Geometry check sheet. Reference: the model listing, model coordinates, mm. Give positions to 0.01 mm unless a question says otherwise; leave off trailing zeros. Loops run counter-clockwise (first coordinate to the right, second up) from the corner with the lowest first, then second, coordinate; pieces in that order, holes last. Notation, with made-up numbers: (66.25, -1) - (94.25, -1) arc R27 ccw to (94.25, 15) - close; hole circle Ø2 at (59.5, 35.5). An arc over 180 degrees is marked (long way). Use a Markdown table: item, result. Add a question column.
1. Depth check by flat-ended pin: P1, Ø1.6, axis at y = 0, z = -1.5, coming from the -X side; P2, Ø0.7, axis at x = -155.5, y = -0.5, coming from the +Z side; P3, Ø1.6, axis at y = 0.5, z = 98, coming from the +X side. Enter the tip coordinate at first touch or a pass-through.
2. Cross-section at B-B on z = 135.5. Enter the section's corners in (x, y).
3. Cross-section at C-C on x = -15. Enter the section's corners in (y, z), and give its area (3 significant figures).
4. Material ranges on L1, parallel to X at y = 0.45, z = 144; L2, parallel to Z at x = -132, y = -0.95; L3, parallel to X at y = 1.35, z = 53, recorded low to high.
5. Cross-section at A-A on y = -0.8. Enter the section's corners in (x, z) (3 decimals).
from build123d import *

# Parameters (mm, degrees)
SKETCH1_W           = 314.32961264
SKETCH1_H           = 3.175
BOSS_EXTRUDE1_DEPTH = 200.60000012
CUT_EXTRUDE2_START  = -3.175
SKETCH5_W           = 2.286
SKETCH5_H           = 86.36
CUT_EXTRUDE2_DEPTH  = 259.030286425
SKETCH3_W           = 80
SKETCH3_H           = 3.175
BOSS_EXTRUDE2_DEPTH = 3.175
LPATTERN2_COUNT     = 2
LPATTERN2_PITCH     = 154.43
BOSS_EXTRUDE3_DEPTH = 3.175


with BuildPart() as part:
    # Sketch1 → Boss-Extrude1 (new body)
    with BuildSketch(Plane.XY):
        Rectangle(SKETCH1_W, SKETCH1_H)
    extrude(amount=BOSS_EXTRUDE1_DEPTH)

    # Sketch5 → Cut-Extrude2 (cut)
    with BuildSketch(Plane(origin=(0, 1.5875, 0), x_dir=(1, 0, 0), z_dir=(0, 1, 0)).offset(CUT_EXTRUDE2_START)):
        with Locations((-156.02180632, -157.42000012)):
            Rectangle(SKETCH5_W, SKETCH5_H)
    cut_extrude2 = extrude(amount=CUT_EXTRUDE2_DEPTH, mode=Mode.SUBTRACT)

    # Mirror1: Cut-Extrude2 across plane
    add(cut_extrude2.mirror(Plane(origin=(0, 0, 0), x_dir=(0, 0, 1), z_dir=(1, 0, 0))), mode=Mode.SUBTRACT)

    # Sketch3 → Boss-Extrude2 (add)
    with BuildSketch(Plane(origin=(0, 0, 0), x_dir=(-1, 0, 0), z_dir=(0, 0, -1))):
        with Locations((-77.16480632, 0)):
            Rectangle(SKETCH3_W, SKETCH3_H)
    boss_extrude2 = extrude(amount=BOSS_EXTRUDE2_DEPTH)

    # LPattern2: Boss-Extrude2 ×2
    with Locations(*[(-i * LPATTERN2_PITCH, 0, 0) for i in range(1, LPATTERN2_COUNT)]):
        add(boss_extrude2)

    # Sketch10 → Boss-Extrude3 (add)
    with BuildSketch(Plane.XZ.offset(1.5875)):
        Polygon((157.16480632, 0), (195.26480632, 0), (157.16480632, 50.8), align=None)
    extrude(amount=-BOSS_EXTRUDE3_DEPTH)


solid = part.part
Values found:
| question | item | result |
|---|---|---|
| 1 | P1 | stops at x = -117.27 |
| 1 | P2 | stops at z = 114.24 |
| 1 | P3 | stops at x = 157.16 |
| 2 | outline | (-154.88, -1.59) - (154.88, -1.59) - (154.88, 1.59) - (-154.88, 1.59) - close |
| 3 | outline | (-1.59, 0) - (1.59, 0) - (1.59, 200.6) - (-1.59, 200.6) - close |
| 3 | area | 637 mm2 |
| 4 | L1 | x = -154.88 to 154.88 |
| 4 | L2 | z = 0 to 200.6 |
| 4 | L3 | x = -157.16 to 157.16 |
| 5 | outline | (-157.165, 0) - (-117.265, 0) - (-117.265, -3.175) - (-37.265, -3.175) - (-37.265, 0) - (37.165, 0) - (37.165, -3.175) - (117.165, -3.175) - (117.165, 0) - (195.265, 0) - (157.165, 50.8) - (157.165, 114.24) - (154.879, 114.24) - (154.879, 200.6) - (-154.879, 200.6) - (-154.879, 114.24) - (-157.165, 114.24) - close |
